Source: CAD feature listing. Evaluate the final solid. Frame: model axes, mm. Face numbers are marked on the shaded views. A direction names the side the tool comes from. Coordinates: 2 decimals unless noted, no trailing zeros. Write each loop counter-clockwise with the first axis right and the second up, starting at its lowest first coordinate (ties: lowest second). Pieces come first, ordered by that corner, then holes. Notation, with made-up numbers: (81.5, 49.5) - (117.5, 49.5) arc R15 cw to (117.5, 75.5) - close; hole circle Ø1 at (46.5, 88). An arc over 180 degrees is marked (long way). One line per item, written item: value.
from build123d import *

# Parameters (mm, degrees)
SCHIZZO1_W                   = 66.6
SCHIZZO1_H                   = 66.6
ESTRUSIONE_ESTRUSIONE1_DEPTH = 3
SCHIZZO2_W                   = 3
SCHIZZO2_H                   = 66.6
ESTRUSIONE_ESTRUSIONE2_DEPTH = 63.6
SCHIZZO6_W                   = 60.6
SCHIZZO6_H                   = 3
ESTRUSIONE_ESTRUSIONE4_DEPTH = 63.6
TAGLIO_ESTRUSIONE2_DEPTH     = 66.6
ESTRUSIONE_ESTRUSIONE5_DEPTH = 63.6
SCHIZZO9_R                   = 6
TAGLIO_ESTRUSIONE4_DEPTH     = 94.9479111


with BuildPart() as part:
    # Schizzo1 → Estrusione-Estrusione1 (new body)
    with BuildSketch(Plane.XY):
        Rectangle(SCHIZZO1_W, SCHIZZO1_H)
    extrude(amount=ESTRUSIONE_ESTRUSIONE1_DEPTH)

    # Schizzo2 → Estrusione-Estrusione2 (add)
    with BuildSketch(Plane.XY.offset(3)):
        with Locations((-31.8, 0)):
            Rectangle(SCHIZZO2_W, SCHIZZO2_H)
        with Locations((31.8, 0)):
            Rectangle(SCHIZZO2_W, SCHIZZO2_H)
    extrude(amount=ESTRUSIONE_ESTRUSIONE2_DEPTH)

    # Schizzo6 → Estrusione-Estrusione4 (add)
    with BuildSketch(Plane.XY.offset(3)):
        with Locations((0, 31.8)):
            Rectangle(SCHIZZO6_W, SCHIZZO6_H)
    extrude(amount=ESTRUSIONE_ESTRUSIONE4_DEPTH)

    # Schizzo7 → Taglio-Estrusione2 (cut)
    with BuildSketch(Plane.XY.offset(66.6)):
        with BuildLine():
            Line((-33.3, 23.3), (-33.3, 33.3))
            Line((-33.3, 33.3), (-23.3, 33.3))
            ThreePointArc((-23.3, 33.3), (-30.371067812, 30.371067812), (-33.3, 23.3))
        make_face()
        with BuildLine():
            Line((33.3, 33.3), (33.3, 23.3))
            ThreePointArc((33.3, 23.3), (30.371067812, 30.371067812), (23.3, 33.3))
            Line((23.3, 33.3), (33.3, 33.3))
        make_face()
    extrude(amount=-TAGLIO_ESTRUSIONE2_DEPTH, mode=Mode.SUBTRACT)

    # Schizzo8 → Estrusione-Estrusione5 (add)
    with BuildSketch(Plane.XY.offset(3)):
        with BuildLine():
            Line((-30.3, 23.3), (-30.3, 30.3))
            Line((-30.3, 30.3), (-23.3, 30.3))
            ThreePointArc((-23.3, 30.3), (-28.249747468, 28.249747468), (-30.3, 23.3))
        make_face()
        with BuildLine():
            Line((30.3, 30.3), (30.3, 23.3))
            ThreePointArc((30.3, 23.3), (28.249747468, 28.249747468), (23.3, 30.3))
            Line((23.3, 30.3), (30.3, 30.3))
        make_face()
    extrude(amount=ESTRUSIONE_ESTRUSIONE5_DEPTH)

    # Schizzo9 → Taglio-Estrusione4 (cut, through all)
    with BuildSketch(Plane(origin=(0, 27.3, 3), x_dir=(1, 0, 0), z_dir=(0, 0, 1))):
        with Locations((0, -14.8)):
            Circle(SCHIZZO9_R)
    extrude(amount=-TAGLIO_ESTRUSIONE4_DEPTH, mode=Mode.SUBTRACT)


solid = part.part
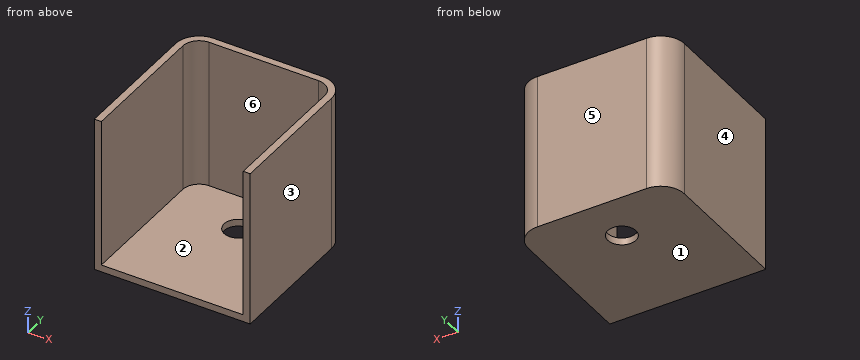
1) Section query A-A on x = 0. Output: boundary loops of the cut face in (y, z), then the cut area to 3 significant figures.
Values found:
outline: (-33.3, 0) - (6.5, 0) - (6.5, 3) - (-33.3, 3) - close; (18.5, 0) - (33.3, 0) - (33.3, 66.6) - (30.3, 66.6) - (30.3, 3) - (18.5, 3) - close
area: 355 mm2
2) Section query D-D on y = -7.5. Output: boundary loops of the cut face in (x, z), then the cut area to 3 significant figures.
Values found:
outline: (-33.3, 0) - (33.3, 0) - (33.3, 66.6) - (30.3, 66.6) - (30.3, 3) - (-30.3, 3) - (-30.3, 66.6) - (-33.3, 66.6) - close
area: 581 mm2
3) Section query C-C on z = 43.5. Output: boundary loops of the cut face in (x, y), then the cut area to 3 significant figures.
Values found:
outline: (-33.3, -33.3) - (-30.3, -33.3) - (-30.3, 23.3) arc R7 cw to (-23.3, 30.3) - (23.3, 30.3) arc R7 cw to (30.3, 23.3) - (30.3, -33.3) - (33.3, -33.3) - (33.3, 23.3) arc R10 ccw to (23.3, 33.3) - (-23.3, 33.3) arc R10 ccw to (-33.3, 23.3) - close
area: 560 mm2
4) Section query B-B on y = 12.5. Output: boundary loops of the cut face in (x, z), then the cut area to 3 significant figures.
Values found:
outline: (-33.3, 0) - (-6, 0) - (-6, 3) - (-30.3, 3) - (-30.3, 66.6) - (-33.3, 66.6) - close; (6, 0) - (33.3, 0) - (33.3, 66.6) - (30.3, 66.6) - (30.3, 3) - (6, 3) - close
area: 545 mm2
5) Contact query for flat-ended pins moving along their axis: P1, Ø6, axis at x = -18.5, y = 10.5, coming from the -Z side; P2, Ø14, axis at x = 5, z = 26, coming from the -Y side; P3, Ø12, axis at x = 12, y = 3.5, coming from the +Z side. Output: stop coordinate, or through.
Values found:
P1: z = 0
P2: y = 30.3
P3: z = 3
6) Reachability of the marked faces 1 and 2 from +Z, -Z, +X, -X, +Y, -Y: full face, straight path, thin tool, end or side. Return the list, or none.
Values found:
face 1: -Z, +X, -X, +Y, -Y
face 2: +Z, -Y
7) Material intervals for line 1 (X direction, y = 12, z = 1); line 2 (X direction, y = 6.5, z = 34); line 3 (Y direction, x = 11, z = 55.5), sorted ascending.
Values found:
line 1: -33.3 to -5.98, 5.98 to 33.3
line 2: -33.3 to -30.3, 30.3 to 33.3
line 3: 30.3 to 33.3
8) Draft query along X for the marked faces 3, 4, 5 and 6. Return one class per face: released by +X, released by -X, zero draft, split by the parting line, or undercut.
Values found:
face 3: released by +X
face 4: released by -X
face 5: zero draft
face 6: undercut
